The listing builds one solid part. Answer for the finished solid, in the listing's coordinates (mm). A direction names the side the tool comes from. Coordinates: 2 decimals unless noted, no trailing zeros. Order: outer loops, then holes, each group sorted by start corner. A loop starts at its lowest first (then second) coordinate and runs counter-clockwise, first axis right, second up. Notation, with made-up numbers: (64, -31.75) -> (84, -31.75) arc R24 ccw to (84, -16.75) -> close; hole circle Ø8 at (74, 78). An arc over 180 degrees is marked (long way). Answer in a Markdown table with one row per item. Add a question column.
```python
from build123d import *

# Parameters (mm, degrees)
RESSALTO_EXTRUS_O1_DEPTH = 3
FILETE1_R                = 25
ESBO_O2_R                = 10
CORTE_EXTRUS_O1_DEPTH    = 556.395887416


with BuildPart() as part:
    # Esboço1 → Ressalto-extrusão1 (new body)
    with BuildSketch(Plane.XY):
        Polygon((-18.228540014, 416.846731975), (-150, 259.807621135), (0, 0), (95, 0), (120, 25), (210, 25), (235, 0), (330, 0), (370, 40), (287.829512447, 182.323459324), (259.709984143, 192.558130628), (169.709984143, 348.44270331), align=None)
        Polygon((0, 0), (-150, 259.807621135), (-18.228540014, 416.846731975), (-23.228540014, 418.666583146), (-156.080645864, 260.339608715), (-2.886751346, -5), (97.071067812, -5), (122.071067812, 20), (207.928932188, 20), (232.928932188, -5), (332.071067812, -5), (376.248444489, 39.177376677), (291.249713881, 186.399496669), (263.130185576, 196.634167974), (177.019495143, 345.782258878), (169.709984143, 348.44270331), (259.709984143, 192.558130628), (287.829512447, 182.323459324), (370, 40), (330, 0), (235, 0), (210, 25), (120, 25), (95, 0), align=None)
    extrude(amount=RESSALTO_EXTRUS_O1_DEPTH)

    # Filete1
    filete1_edges = [part.edges().sort_by_distance(p)[0] for p in [
        (177.019495143, 345.782258878, 1.5),
        (263.130185576, 196.634167974, 1.5),
        (291.249713881, 186.399496669, 1.5),
        (376.248444489, 39.177376677, 1.5),
        (332.071067812, -5, 1.5),
        (232.928932188, -5, 1.5),
        (207.928932188, 20, 1.5),
        (122.071067812, 20, 1.5),
        (97.071067812, -5, 1.5),
        (-2.886751346, -5, 1.5),
        (-156.080645864, 260.339608715, 1.5),
        (-23.228540014, 418.666583146, 1.5),
    ]]
    fillet(filete1_edges, radius=FILETE1_R)

    # Esboço2 → Corte-extrusão1 (cut, through all)
    with BuildSketch(Plane(origin=(0, 0, 0), x_dir=(-1, 0, 0), z_dir=(0, 0, -1))):
        with Locations((11.909345747, 393.263177907)):
            Circle(ESBO_O2_R)
        with Locations((125.677416542, 257.679670815)):
            Circle(ESBO_O2_R)
        with Locations((-48.61042611, 20)):
            Circle(ESBO_O2_R)
        with Locations((-320.673846837, 20)):
            Circle(ESBO_O2_R)
        with Locations((-285.673846837, 161.319502665)):
            Circle(ESBO_O2_R)
    extrude(amount=-CORTE_EXTRUS_O1_DEPTH, mode=Mode.SUBTRACT)


solid = part.part
```
Q1. Straight lines are drawn through the part: line 1 (X direction, y = 24.5, z = 0.7); line 2 (Y direction, x = 168.5, z = 1.25); line 3 (Y direction, x = 74, z = 1.9). For each, find the intervals that lie inside material, in ascending order.
Q2. For faces 1 (the face through (82.07, 380.34, 1.48)), 2 (the face through (220.36, 7.57, 1.48)), determine the directions among +Z, -Z, +X, -X, +Y, -Y from which every point of the face is accessible in a straight line to the end or side of a thin tool.
Q3. Determine the mould class of faces 3 (the face through (220.6, 270.3, 1.5)), 4 (the face through (106, 161, 0)), 5 (the face through (-88.9, 340.4, 1.5)), 6 (the face through (49.912, 29.915, 1.479)) for opening direction X: +X half, -X half, draft (parallel to the pull), parting line (faces both ways), or undercut.
Q4. A cutting plane is placed at B-B (x = 191). Determine the outline of the cut face in (y, z).
Q5. A cutting plane is placed at A-A (z = 1.7). State how many separate pieces and enclosed holes the cut face has, then the cut area to 3 significant figures.
Q6. Given pin 1 (8 mm diameter, centred on x = 153.5, y = 93.5, fed in from -Z); pin 2 (1.5 mm diameter, centred on x = 156.5, z = 0.5, fed in from +Y), each flat-ended and moving along its own axis, determine where each tip first touches the part or whether it passes through.
Q7. A cutting plane is placed at C-C (y = 75). Determine the outline of the cut face in (x, z).
Returned:
| question | item | result |
|---|---|---|
| 1 | line 1 | x = -19.92 to 39.68, 57.54 to 311.74, 329.6 to 361.57 |
| 1 | line 2 | y = 20 to 348.88 |
| 1 | line 3 | y = -5 to 383.28 |
| 2 | face 1 | +Z, -Z, +X, +Y |
| 2 | face 2 | +Z, -Z, -Y |
| 3 | face 3 | +X half |
| 3 | face 4 | draft |
| 3 | face 5 | -X half |
| 3 | face 6 | undercut |
| 4 | outline | (20, 0) -> (321.57, 0) -> (321.57, 3) -> (20, 3) -> close |
| 5 | separate pieces | 1 |
| 5 | enclosed holes | 5 |
| 5 | area | 137,000 mm² |
| 6 | pin 1 | stops at z = 0 |
| 6 | pin 2 | stops at y = 353.52 |
| 7 | outline | (-49.07, 0) -> (355.57, 0) -> (355.57, 3) -> (-49.07, 3) -> close |
